from build123d import *

# Parameters (mm, degrees)
F1_DEPTH = 1.6
F3_D     = 3
F5_D     = 6.5


with BuildPart() as f1:
    # F0 (on Top) → F1 (new body)
    with BuildSketch(Plane.XY):
        with BuildLine():
            Line((-20, 52), (-20, 48))
            ThreePointArc((-20, 48), (0, -52), (20, 48))
            Line((20, 48), (20, 52))
            Line((20, 52), (-20, 52))
        make_face()
    extrude(amount=F1_DEPTH)

    # F3 (through all)
    with Locations(Plane.XY.offset(1.6)):
        with Locations((-22, 43.783559), (22, 43.783559), (42.435245, -24.5), (-42.435245, -24.5)):
            Hole(F3_D / 2)

    # F5 (through all)
    with Locations(Plane.XY.offset(1.6)):
        with Locations((0, 0)):
            Hole(F5_D / 2)


solid = f1.part
Here's how the part is built. I have some questions about the finished solid (model axes, mm). Give positions to 0.01 mm unless a question says otherwise; leave off trailing zeros. Loops run counter-clockwise (first coordinate to the right, second up) from the corner with the lowest first, then second, coordinate; pieces in that order, holes last. Notation, with made-up numbers: (-25.75, 46) -> (-14.75, 46) arc R5 cw to (-14.75, 55) -> close; hole circle Ø7 at (71, -7.5). An arc over 180 degrees is marked (long way). One line per item, written item: value.
Q1. Suppose I cut it at A-A on y = 0. Please give me the cut outline in (x, z), then the cut area to 3 significant figures.
Answers follow:
outline: (-52, 0) -> (-3.25, 0) -> (-3.25, 1.6) -> (-52, 1.6) -> close; (3.25, 0) -> (52, 0) -> (52, 1.6) -> (3.25, 1.6) -> close
area: 156 mm^2
Q2. I'm going to push flat-ended pins straight in: pin 1 Ø0.8 at (y, z) = (50, 0.5) entering from -X; pin 2 Ø0.8 at (y, z) = (49.5, 0.5) entering from +X; pin 3 Ø4 at (x, y) = (0, 0) entering from +Z. Where does each tip first touch, or does it pass through?
Answers follow:
pin 1: x = -20
pin 2: x = 20
pin 3: through
Q3. Suppose I cut it at D-D on z = 0.6. Please give me the cut outline in (x, y).
Answers follow:
outline: (-20, 48) arc R52 ccw (long way) to (20, 48) -> (20, 52) -> (-20, 52) -> close; hole circle Ø3 at (-42.44, -24.5); hole circle Ø3 at (-22, 43.78); hole circle Ø6.5 at (0, 0); hole circle Ø3 at (22, 43.78); hole circle Ø3 at (42.44, -24.5)
Q4. If I drill on line 1 along Y through (x, z) = (22, 0.85); line 2 along X through (y, z) = (-2, 0.6); line 3 along X through (y, z) = (-45.5, 1.45), over which ranges is the centre line in solid material (lowest first)?
Answers follow:
line 1: -47.12 to 42.28, 45.28 to 47.12
line 2: -51.96 to -2.56, 2.56 to 51.96
line 3: -25.17 to 25.17
Q5. Suppose I cut it at C-C on y = -24.5. Please give me the cut outline in (x, z), then the cut area to 3 significant figures.
Answers follow:
outline: (-45.87, 0) -> (-43.94, 0) -> (-43.94, 1.6) -> (-45.87, 1.6) -> close; (-40.94, 0) -> (40.94, 0) -> (40.94, 1.6) -> (-40.94, 1.6) -> close; (43.94, 0) -> (45.87, 0) -> (45.87, 1.6) -> (43.94, 1.6) -> close
area: 137 mm^2
Q6. We'd pull the mould along X, two halves only. Please class faces 1 (the face through (11, 1, 1.6)), 2 (the face through (-2, -51.96, 0.79)), 3 (the face through (23.106, 44.797, 0.789)), 4 (the face through (-20.894, 44.797, 0.789)): pulls with the +X half, pulls with the -X half, needs draft (parallel to the pull), parting line crosses it, or undercut.
Answers follow:
face 1: needs draft
face 2: parting line crosses it
face 3: undercut
face 4: undercut
